Source: three-view drawing plus pictorial views. Frame: mm from the lowest corner of the part. A direction names the side the tool comes from. Give positions to 0.01 mm unless a question says otherwise; leave off trailing zeros. Loops run counter-clockwise (first coordinate to the right, second up) from the corner with the lowest first, then second, coordinate; pieces in that order, holes last.
1. Section B-B, the plane x = 59. Output: boundary loops of the cut face in (y, z).
2. Section A-A, the plane y = 15. Output: boundary loops of the cut face in (x, z), then the cut area to 3 significant figures.
3. Access query for the marked faces 1 and 2. Directions: +Z, -Z, +X, -X, +Y, -Y. A direction counts if a zero-diameter tool reaches every point of the face in a straight line with its end or side. Return the directions, or none.
4. Section D-D, the plane y = 45. Output: boundary loops of the cut face in (x, z).
5. First-contact query: P1, Ø4, axis at x = 45, y = 46, coming from the +Z side; P2, Ø10, axis at y = 52.5, z = 7.5, coming from the -X side; P3, Ø6.5, axis at x = 16, y = 46, coming from the -Z side; P4, Ø10, axis at x = 130, y = 24, coming from the +Z side. Flat tips, straight axial feed; report the tip coordinate or a pass-through.
6. Section C-C, the plane z = 35. Output: boundary loops of the cut face in (x, y).
7. Draft query along Z for the marked faces 3, 4, 5 and 6. Return one class per face: +Z half, -Z half, draft (parallel to the pull), parting line (faces both ways), or undercut.
8. Material intervals for line 1 along X through (y, z) = (5, 25.5); line 2 along Z through (x, y) = (14.5, 35); line 3 along Z through (x, y) = (58.5, 56), sorted ascending.
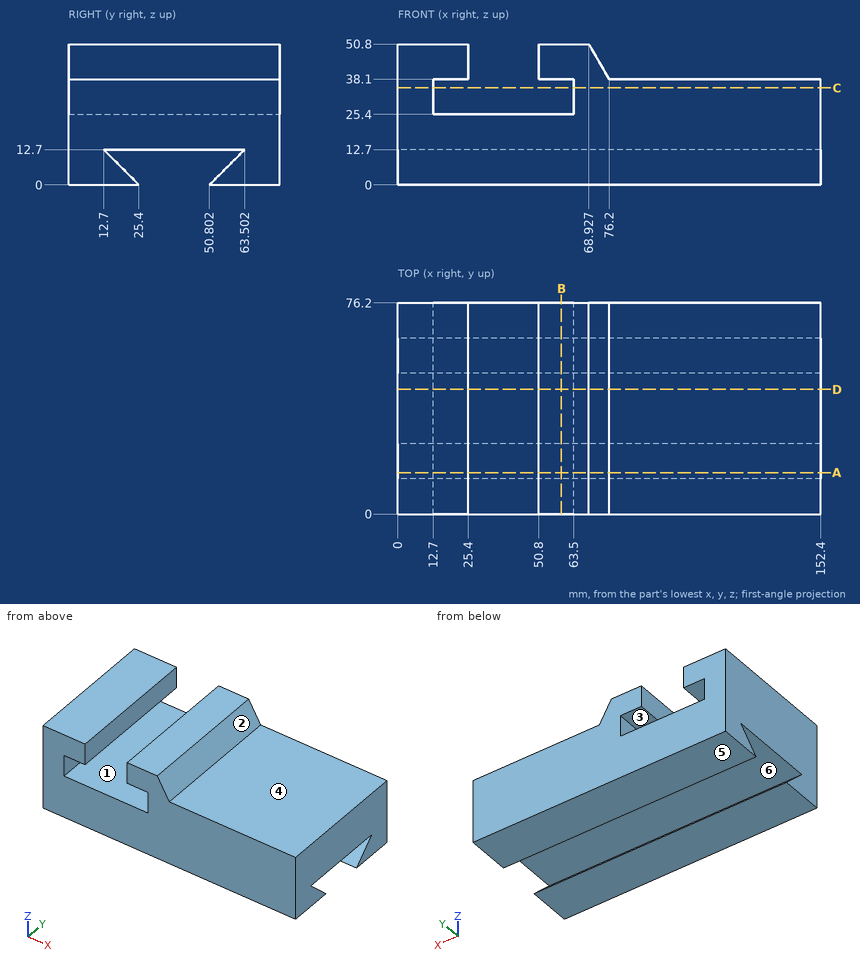
Answers below:
1. outline: (0, 0) - (25.4, 0) - (12.7, 12.7) - (63.5, 12.7) - (50.8, 0) - (76.2, 0) - (76.2, 25.4) - (0, 25.4) - close; (0, 38.1) - (76.2, 38.1) - (76.2, 50.8) - (0, 50.8) - close
2. outline: (0, 0) - (152.4, 0) - (152.4, 10.4) - (0, 10.4) - close; (0, 12.7) - (152.4, 12.7) - (152.4, 38.1) - (76.2, 38.1) - (68.93, 50.8) - (50.8, 50.8) - (50.8, 38.1) - (63.5, 38.1) - (63.5, 25.4) - (12.7, 25.4) - (12.7, 38.1) - (25.4, 38.1) - (25.4, 50.8) - (0, 50.8) - close
2. area: 5,410 mm2
3. face 1: +Y, -Y
3. face 2: +Z, +X, +Y, -Y
4. outline: (0, 12.7) - (152.4, 12.7) - (152.4, 38.1) - (76.2, 38.1) - (68.93, 50.8) - (50.8, 50.8) - (50.8, 38.1) - (63.5, 38.1) - (63.5, 25.4) - (12.7, 25.4) - (12.7, 38.1) - (25.4, 38.1) - (25.4, 50.8) - (0, 50.8) - close
5. P1: stops at z = 25.4
5. P2: stops at x = 0
5. P3: stops at z = 12.7
5. P4: stops at z = 38.1
6. outline: (0, 0) - (12.7, 0) - (12.7, 76.2) - (0, 76.2) - close; (63.5, 0) - (152.4, 0) - (152.4, 76.2) - (63.5, 76.2) - close
7. face 3: undercut
7. face 4: +Z half
7. face 5: -Z half
7. face 6: undercut
8. line 1: x = 0 to 12.7, 63.5 to 152.4
8. line 2: z = 12.7 to 25.4, 38.1 to 50.8
8. line 3: z = 0 to 5.2, 12.7 to 25.4, 38.1 to 50.8
